Part model, mm, in its own coordinate system. Face numbers are marked on the shaded views. A direction names the side the tool comes from. Coordinates: 2 decimals unless noted, no trailing zeros. Loops run counter-clockwise (first coordinate to the right, second up) from the corner with the lowest first, then second, coordinate; pieces in that order, holes last. Notation, with made-up numbers: (-37, -34) - (0, -34) arc R28 cw to (0, -3) - close; hole circle Ø2 at (13, 49). An arc over 180 degrees is marked (long way). Use a Markdown table: item, result. Add a question column.
1) Band-saw the part on C-C (z = -2.5). Give the cut face in (x, y) (3 decimals), plus the area to 3 significant figures.
2) Band-saw the part on A-A (y = -4.5). Give the number of separate pieces and of enclosed holes in the cut face, plus the area to 3 significant figures.
3) Tool access for the marked faces 4 and 5: list every direction of +Z, -Z, +X, -X, +Y, -Y with a clear straight run to the whole face (end or side of a thin tool).
4) Drop flat-ended pins along their axis: P1, Ø2, axis at y = -8, z = -6, coming from the +X side; P2, Ø5, axis at x = -4.5, y = -10, coming from the +Z side; P3, Ø3, axis at x = -2, y = -2, coming from the -Z side. Give the stop position or say it passes through.
5) Pull direction Z, two halves, no side cores. Call the marked faces 1, 2 and 3: +Z half, -Z half, draft (parallel to the pull), parting line (faces both ways), or undercut.
6) Probe probe 1 along Z at (x, y) = (19, -3.75); probe 2 along X at (y, z) = (-10.75, -11.5); probe 3 along X at (y, z) = (-8.5, 1.5). List the from-to ranges inside material, lowest first. Write a range as [from, to].
7) Band-saw the part on D-D (z = -12). Give the cut face in (x, y), plus the area to 3 significant figures.
8) Band-saw the part on B-B (x = -12). Give the cut face in (y, z), plus the area to 3 significant figures.
from build123d import *

# Parameters (mm, degrees)
F0_R     = 27.5
F0_R_2   = 23.5
F1_DEPTH = 12
F2_R     = 27.467617
F3_DEPTH = 0.254
F4_R     = 3.5
F4_R_2   = 2.5
F4_R_3   = 1.5
F5_DEPTH = 12
F7_DEPTH = 12
F9_DEPTH = 12


with BuildPart() as f1:
    # F0 (on Front) → F1 (new body)
    with BuildSketch(Plane.XZ):
        Circle(F0_R)
        Circle(F0_R_2, mode=Mode.SUBTRACT)
    extrude(amount=F1_DEPTH)

    # F2 (on Front) → F3 (join)
    with BuildSketch(Plane.XZ):
        Circle(F2_R)
    extrude(amount=F3_DEPTH)

    # F4 (on Front) → F5 (join)
    with BuildSketch(Plane.XZ):
        with Locations((17.688596, 0.011209)):
            Circle(F4_R)
        with Locations((-17.700713, 0)):
            Circle(F4_R)
        with Locations((-13.821965, 9.565342)):
            Circle(F4_R_2)
        with Locations((-8.427355, 15.38721)):
            Circle(F4_R_3)
        with Locations((9.352645, 15.305277)):
            Circle(F4_R_3)
        with Locations((14.118035, 9.117616)):
            Circle(F4_R_2)
    extrude(amount=F5_DEPTH)

    # F6 (on Front) → F7 (join)
    with BuildSketch(Plane.XZ):
        Polygon((4.064, 4.721983), (0, 12.913237), (-3.977783, 4.721983), (-1.988892, 4.721983), (0, 8.81761), (2.032, 4.721983), align=None)
        Polygon((-0.554775, 9.738115), (0, 10.880535), (0.554775, 9.738115), align=None, mode=Mode.SUBTRACT)
        Polygon((0, -4.619357), (-3.977783, 0), (-3.977783, -9.144), (-1.988892, -9.144), (-1.988892, -5.041345), (0, -6.754003), (1.988892, -5.041345), (1.988892, -9.144), (3.977783, -9.144), (3.977783, 0), align=None)
    extrude(amount=F7_DEPTH)

    # F8 (on Front) → F9 (join)
    with BuildSketch(Plane.XZ):
        Polygon((-10.213404, -10.713155), (-12.727875, -8.198683), (-15.242347, -10.713155), (-12.727875, -13.227626), align=None)
        Polygon((12.727869, -8.198683), (10.213398, -10.713155), (12.727869, -13.227626), (15.242341, -10.713155), align=None)
        Polygon((1.725041, -19.36011), (0, -17.221719), (-1.635694, -19.36011), (0, -21.498501), align=None)
    extrude(amount=F9_DEPTH)


solid = f1.part
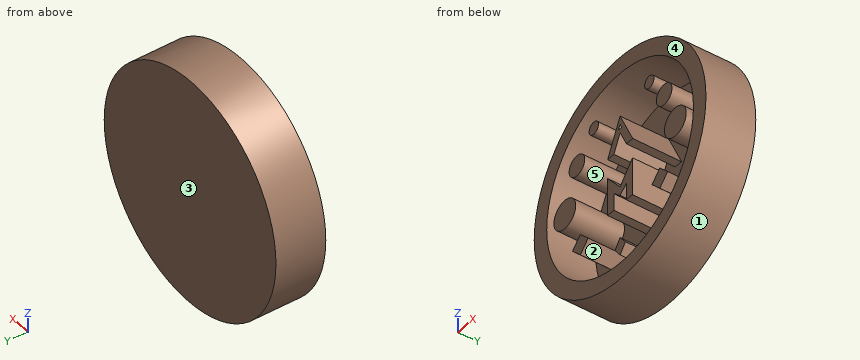
Answer block:
| question | item | result |
|---|---|---|
| 1 | outline | (-27.386, -12) - (-23.367, -12) - (-23.367, -0.254) - (-20.15, -0.254) - (-20.15, -12) - (-15.251, -12) - (-15.251, -0.254) - (-3.978, -0.254) - (-3.978, -12) - (-1.825, -12) - (-1.825, -0.254) - (1.825, -0.254) - (1.825, -12) - (3.978, -12) - (3.978, -0.254) - (15.251, -0.254) - (15.251, -12) - (20.127, -12) - (20.127, -0.254) - (23.367, -0.254) - (23.367, -12) - (27.386, -12) - (27.386, 0) - (-27.386, 0) - close |
| 1 | area | 274 mm2 |
| 2 | separate pieces | 12 |
| 2 | enclosed holes | 2 |
| 2 | area | 869 mm2 |
| 3 | face 4 | +Z, -Z, +X, -X, -Y |
| 3 | face 5 | -Y |
| 4 | P1 | x = 27.04 |
| 4 | P2 | z = 27.43 |
| 4 | P3 | z = -27.5 |
| 5 | face 1 | parting line |
| 5 | face 2 | undercut |
| 5 | face 3 | draft |
| 6 | probe 1 | [-19.88, -13.83], [-3.23, 3.26], [13.83, 19.88] |
| 6 | probe 2 | [-24.98, -20.49], [-14.46, -11], [11, 14.46], [20.49, 24.98] |
| 6 | probe 3 | [-27.46, -23.45], [-20.86, -14.54], [14.52, 20.86], [23.45, 27.46] |
| 7 | outline | (-24.74, -12) - (-20.21, -12) - (-20.21, -0.25) - (-13.96, -0.25) - (-13.96, -12) - (-11.5, -12) - (-11.5, -0.25) - (11.5, -0.25) - (11.5, -12) - (13.96, -12) - (13.96, -0.25) - (20.21, -0.25) - (20.21, -12) - (24.74, -12) - (24.74, 0) - (-24.74, 0) - close |
| 7 | area | 177 mm2 |
| 8 | outline | (-12, -24.74) - (0, -24.74) - (0, 24.74) - (-12, 24.74) - (-12, 20.21) - (-0.25, 20.21) - (-0.25, 11.28) - (-12, 11.28) - (-12, 7.85) - (-0.25, 7.85) - (-0.25, -8.93) - (-12, -8.93) - (-12, -12.5) - (-0.25, -12.5) - (-0.25, -20.21) - (-12, -20.21) - close |
| 8 | area | 201 mm2 |
